The model under review builds one solid part; all positions refer to its coordinate system, in mm. A direction names the side the tool comes from. Give positions to 0.01 mm unless a question says otherwise; leave off trailing zeros. Order: outer loops, then holes, each group sorted by start corner. A loop starts at its lowest first (then second) coordinate and runs counter-clockwise, first axis right, second up. Notation, with made-up numbers: (-13.75, 66) - (38.25, 66) arc R30 ccw to (38.25, 100) - close; hole circle Ø10 at (73.25, 63.5). An arc over 180 degrees is marked (long way). Use CSV: the item, a comma, the result in double quotes. Start each with the question number.
1. Take a section at D-D, the plane y = 50. State the section outline as (x, z) points, then the cut area to 3 significant figures.
2. To check wall thickness, follow line 1 (X direction, y = 96, z = 0); line 2 (Y direction, x = 39, z = -47.5); line 3 (Y direction, x = -39, z = -8). State the ranges of each line that lie inside material, in increasing order. Write a range as [from, to].
3. Draft analysis for pull direction Z (two halves, no side actions). For faces 1 (the cylindrical face through (-103.692, 95.07, -0.346)), 2 (the flat face through (-65.074, 95.07, -20.173)), 3 (the cylindrical face through (-96.214, 4.93, -0.976)), state which applies: released by +Z, released by -Z, zero draft, split by the parting line, or undercut.
4. Take a section at C-C, the plane z = -20. State the section outline as (x, y) points.
5. Take a section at B-B, the plane x = -26. State the section outline as (y, z) points.
6. For pin 1 (5 mm diameter, centred on y = 19.5, z = 37.5, fed in from +X); pin 2 (1.5 mm diameter, centred on y = 51, z = -18.5, fed in from -X); pin 3 (12 mm diameter, centred on y = 50.5, z = -27, fed in from -X), all flat-tipped, find the tip position at first contact; note any pin that passes through.
7. Machinability: for faces 4 (the flat face through (50.165, 95.07, 46.901)), 5 (the flat face through (36, 90, 58)), 6 (the cylindrical face through (51.586, 95.07, 90.045)), which of the approach directions +Z, -Z, +X, -X, +Y, -Y give a long, thin tool a straight path to every point of the face, cutting with its end or side? Answer none if there is none.
8. Take a section at A-A, the plane z = 0. State the section outline as (x, y) points.
```python
from build123d import *

# Parameters (mm, degrees)
SKETCH1_R            = 50
SKETCH1_R_2          = 40
BOSS_EXTRUDE2_DEPTH  = 100
SKETCH4_R            = 40
SKETCH4_R_2          = 30
BOSS_EXTRUDE5_DEPTH  = 5
SKETCH2_R            = 40
BOSS_EXTRUDE6_DEPTH  = 5
SKETCH5_R            = 35
CUT_EXTRUDE1_DEPTH   = 5
SKETCH8_R            = 15
SKETCH8_R_2          = 7.5
SKETCH8_R_3          = 14.918013771
BOSS_EXTRUDE9_DEPTH  = 10
BOSS_EXTRUDE13_DEPTH = 10
SKETCH18_R           = 7.5
CUT_EXTRUDE5_DEPTH   = 10


with BuildPart() as part:
    # Sketch1 → Boss-Extrude2 (new body)
    with BuildSketch(Plane(origin=(0, 0, 0), x_dir=(1, 0, 0), z_dir=(0, 1, 0))):
        with Locations(Location((0, 0, 0), (0, 0, 270))):
            Circle(SKETCH1_R)
        with Locations(Location((0, 0, 0), (0, 0, 270))):
            Circle(SKETCH1_R_2, mode=Mode.SUBTRACT)
    extrude(amount=BOSS_EXTRUDE2_DEPTH)

    # Sketch4 → Boss-Extrude5 (add)
    with BuildSketch(Plane(origin=(0, 100, 0), x_dir=(1, 0, 0), z_dir=(0, 1, 0))):
        with Locations(Location((0, 0, 0), (0, 0, 270))):
            Circle(SKETCH4_R)
        with Locations(Location((0, 0, 0), (0, 0, 270))):
            Circle(SKETCH4_R_2, mode=Mode.SUBTRACT)
    extrude(amount=-BOSS_EXTRUDE5_DEPTH)

    # Sketch2 → Boss-Extrude6 (add)
    with BuildSketch(Plane(origin=(0, 0, 0), x_dir=(1, 0, 0), z_dir=(0, 1, 0))):
        with Locations(Location((0, 0, 0), (0, 0, 270))):
            Circle(SKETCH2_R)
    extrude(amount=BOSS_EXTRUDE6_DEPTH)

    # Sketch5 → Cut-Extrude1 (cut)
    with BuildSketch(Plane.XZ):
        with Locations(Location((0, 0, 0), (0, 0, 270))):
            Circle(SKETCH5_R)
    extrude(amount=-CUT_EXTRUDE1_DEPTH, mode=Mode.SUBTRACT)

    # Sketch8 → Boss-Extrude9 (add)
    with BuildSketch(Plane(origin=(0, 100, 0), x_dir=(1, 0, 0), z_dir=(0, 1, 0))):
        with BuildLine():
            ThreePointArc((-43.301270189, -25), (-50, 0), (-43.301270189, 25))
            Line((-43.301270189, 25), (-87.465711201, 15.208979149))
            ThreePointArc((-87.465711201, 15.208979149), (-87.49541557, 15.037151885), (-87.524782384, 14.865266608))
            ThreePointArc((-87.524782384, 14.865266608), (-77.795338999, 10.095768004), (-73.860157435, 0))
            ThreePointArc((-73.860157435, 0), (-77.795338999, -10.095768004), (-87.524782384, -14.865266608))
            ThreePointArc((-87.524782384, -14.865266608), (-87.49541557, -15.037151885), (-87.465711201, -15.208979149))
            Line((-87.465711201, -15.208979149), (-43.301270189, -25))
        make_face()
        with BuildLine():
            ThreePointArc((0, 50), (24.918582465, 43.348174678), (43.207002617, 25.162569917))
            Line((43.207002617, 25.162569917), (57.131969376, 69.588086322))
            ThreePointArc((57.131969376, 69.588086322), (36.661274001, 64.024757205), (31.097944884, 84.49545258))
            Line((31.097944884, 84.49545258), (0, 50))
        make_face()
        with Locations((44.11495713, 77.041769451)):
            Circle(SKETCH8_R)
        with Locations(Location((44.11495713, 77.041769451, 0), (0, 0, 270))):
            Circle(SKETCH8_R_2, mode=Mode.SUBTRACT)
        with Locations((44.389085603, -76.884151566)):
            Circle(SKETCH8_R)
        with Locations(Location((44.389085603, -76.884151566, 0), (0, 0, 270))):
            Circle(SKETCH8_R_2, mode=Mode.SUBTRACT)
        with BuildLine():
            Line((56.839616952, -68.196932683), (43.301270189, -25))
            ThreePointArc((43.301270189, -25), (25, -43.301270189), (0, -50))
            Line((0, -50), (30.482572388, -83.380911864))
            ThreePointArc((30.482572388, -83.380911864), (30.64711663, -83.32057324), (30.811541435, -83.259909903))
            ThreePointArc((30.811541435, -83.259909903), (36.889085603, -63.893770509), (56.699426375, -68.313532564))
            ThreePointArc((56.699426375, -68.313532564), (56.7695516, -68.255268616), (56.839616952, -68.196932683))
        make_face()
        with Locations((-88.778171206, 0)):
            Circle(SKETCH8_R_3)
        with Locations(Location((-88.778171206, 0, 0), (0, 0, 270))):
            Circle(SKETCH8_R_2, mode=Mode.SUBTRACT)
    extrude(amount=-BOSS_EXTRUDE9_DEPTH)

    # Sketch17 → Boss-Extrude13 (add)
    with BuildSketch(Plane(origin=(0, 0, 0), x_dir=(-1, 0, 0), z_dir=(0, -1, 0))):
        with BuildLine():
            Line((43.301270189, -25), (88.778171206, -14.918013771))
            ThreePointArc((88.778171206, -14.918013771), (103.682992353, 0.627249114), (87.524782384, 14.865266608))
            Line((87.524782384, 14.865266608), (43.207002617, 25.162569917))
            ThreePointArc((43.207002617, 25.162569917), (49.999911712, 0.093961898), (43.301270189, -25))
        make_face()
        with BuildLine():
            ThreePointArc((-43.207002617, 25.162569917), (-24.918582465, 43.348174678), (0, 50))
            Line((0, 50), (-31.097944884, 84.49545258))
            ThreePointArc((-31.097944884, 84.49545258), (-51.568640259, 90.058781697), (-57.131969376, 69.588086322))
            Line((-57.131969376, 69.588086322), (-43.207002617, 25.162569917))
        make_face()
        with BuildLine():
            Line((-30.426057059, -82.843793895), (0, -50))
            ThreePointArc((0, -50), (-25, -43.301270189), (-43.301270189, -25))
            Line((-43.301270189, -25), (-56.839616952, -68.196932683))
            ThreePointArc((-56.839616952, -68.196932683), (-51.75145939, -90.161160078), (-30.426057059, -82.843793895))
        make_face()
    extrude(amount=-BOSS_EXTRUDE13_DEPTH)

    # Sketch18 → Cut-Extrude5 (cut)
    with BuildSketch(Plane.XZ):
        with Locations(Location((-88.778171206, 0, 0), (0, 0, 90))):
            Circle(SKETCH18_R)
        with Locations(Location((44.389085603, 76.884151566, 0), (0, 0, 90))):
            Circle(SKETCH18_R)
        with Locations(Location((44.11495713, -77.041769451, 0), (0, 0, 90))):
            Circle(SKETCH18_R)
    extrude(amount=-CUT_EXTRUDE5_DEPTH, mode=Mode.SUBTRACT)


solid = part.part
```
Determined:
1,outline,"circle Ø100 at (0, 0); hole circle Ø80 at (0, 0)"
1,area,"2,830 mm²"
2,line 1,"x = [-103.7, -96.28], [-81.28, -30], [30, 50]"
2,line 2,"y = [0, 10], [90, 100]"
2,line 3,"y = [0, 5], [95, 100]"
3,face 1,"split by the parting line"
3,face 2,"released by -Z"
3,face 3,"undercut"
4,outline,"(-65.85, 90) - (-45.83, 90) - (-45.83, 10) - (-65.43, 10) - (-65.43, 0) - (-28.72, 0) - (-28.72, 5) - (-34.64, 5) - (-34.64, 95) - (-22.36, 95) - (-22.36, 100) - (-65.85, 100) - close; (22.36, 95) - (34.64, 95) - (34.64, 5) - (28.72, 5) - (28.72, 0) - (45.83, 0) - (45.83, 100) - (22.36, 100) - close"
5,outline,"(0, -42.71) - (100, -42.71) - (100, -14.97) - (95, -14.97) - (95, -30.4) - (5, -30.4) - (5, -23.43) - (0, -23.43) - close; (0, 23.43) - (5, 23.43) - (5, 30.4) - (95, 30.4) - (95, 14.97) - (100, 14.97) - (100, 42.71) - (0, 42.71) - close"
6,pin 1,"stops at x = 35.71"
6,pin 2,"stops at x = -46.74"
6,pin 3,"stops at x = -45.38"
7,face 4,"+X, +Y, -Y"
7,face 5,"+Z, +X"
7,face 6,"+Y"
8,outline,"(-103.7, 0) - (-96.28, 0) - (-96.28, 10) - (-103.7, 10) - close; (-103.7, 90) - (-96.28, 90) - (-96.28, 100) - (-103.7, 100) - close; (-81.28, 0) - (-35, 0) - (-35, 5) - (-40, 5) - (-40, 95) - (-30, 95) - (-30, 100) - (-81.28, 100) - (-81.28, 90) - (-50, 90) - (-50, 10) - (-81.28, 10) - close; (30, 95) - (40, 95) - (40, 5) - (35, 5) - (35, 0) - (50, 0) - (50, 100) - (30, 100) - close"
